For this review, take the finished solid that the model builds, in its own axes (mm). Face numbers are marked on the shaded views. A direction names the side the tool comes from. Give positions to 0.01 mm unless a question says otherwise; leave off trailing zeros. Order: outer loops, then holes, each group sorted by start corner. A loop starts at its lowest first (then second) coordinate and runs counter-clockwise, first axis right, second up.
from build123d import *

# Parameters (mm, degrees)
SKETCH_1_R               = 25
SKETCH_1_R_2             = 8
EXTRUDE_1_DEPTH          = 5
SKETCH_2_R               = 11
SKETCH_2_R_2             = 8
EXTRUDE_2_DEPTH          = 5
SKETCH_3_W               = 2
SKETCH_3_H               = 6
CUT_EXTRUDE_1_DEPTH      = 5
PATTERN_CIRCULAR_1_COUNT = 20


with BuildPart() as part:
    # 草图1 → 凸台-拉伸1 (new body)
    with BuildSketch(Plane.XY):
        Circle(SKETCH_1_R)
        Circle(SKETCH_1_R_2, mode=Mode.SUBTRACT)
    extrude(amount=EXTRUDE_1_DEPTH)

    # 草图2 → 凸台-拉伸2 (add)
    with BuildSketch(Plane.XY.offset(5)):
        Circle(SKETCH_2_R)
        Circle(SKETCH_2_R_2, mode=Mode.SUBTRACT)
    extrude(amount=EXTRUDE_2_DEPTH)

    # 草图3 → 切除-拉伸1 (cut)
    with BuildSketch(Plane.XY.offset(5)):
        with Locations((0, 19)):
            Rectangle(SKETCH_3_W, SKETCH_3_H)
    cut_extrude_1 = extrude(amount=-CUT_EXTRUDE_1_DEPTH, mode=Mode.SUBTRACT)

    # 阵列(圆周)1: 切除-拉伸1 ×20 about axis
    pattern_circular_1_axis = Axis((0, 0, 0), (0, 0, 1))
    for i in range(1, PATTERN_CIRCULAR_1_COUNT):
        add(cut_extrude_1.rotate(pattern_circular_1_axis, i * 360 / PATTERN_CIRCULAR_1_COUNT), mode=Mode.SUBTRACT)


solid = part.part
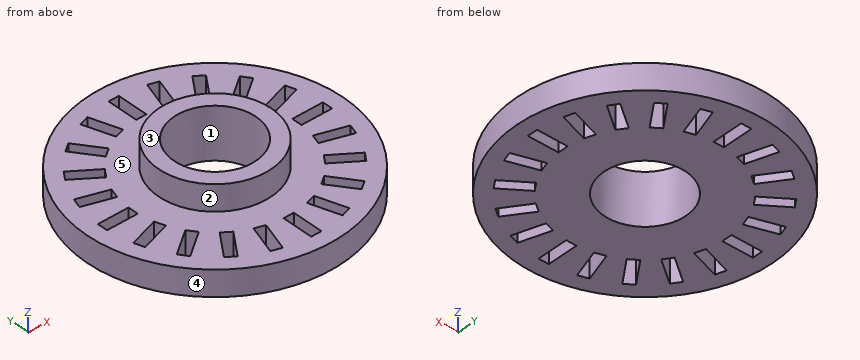
1) Draft analysis for pull direction X (two halves, no side actions). For the marked faces 1, 2 and 3, state which applies: +X half, -X half, draft (parallel to the pull), parting line (faces both ways), or undercut.
Answer sheet:
face 1: undercut
face 2: parting line
face 3: draft
2) Tool access review of the marked faces 4 and 5: name each direction out of +Z, -Z, +X, -X, +Y, -Y from which nothing blocks a thin tool from reaching the whole face with its end or side.
Answer sheet:
face 4: +Z, -Z
face 5: +Z
3) We need section A-A on y = 0. Give the boundary of the cut face in (x, z).
Answer sheet:
outline: (-25, 0) - (-22, 0) - (-22, 5) - (-25, 5) - close; (-16, 0) - (-8, 0) - (-8, 10) - (-11, 10) - (-11, 5) - (-16, 5) - close; (8, 0) - (16, 0) - (16, 5) - (11, 5) - (11, 10) - (8, 10) - close; (22, 0) - (25, 0) - (25, 5) - (22, 5) - close
4) To check wall thickness, follow line 1 (Y direction, x = 0, z = 4.75); line 2 (Y direction, x = 0, z = 7); line 3 (Y direction, x = -10, z = 4.75). State the ranges of each line that lie inside material, in increasing order.
Answer sheet:
line 1: y = -25 to -22, -16 to -8, 8 to 16, 22 to 25
line 2: y = -11 to -8, 8 to 11
line 3: y = -22.91 to -15.47, -12.51 to 12.51, 15.47 to 22.91
5) We need section C-C on z = 8.75. Give the boundary of the cut face in (x, y), then the cut area to 3 significant figures.
Answer sheet:
outline: circle Ø22 at (0, 0); hole circle Ø16 at (0, 0)
area: 179 mm2
6) Clearance check with flat-ended pins moving along their axes: pin 1 (1.5 mm diameter, centred on y = -20, z = 3, fed in from -X); pin 2 (1.6 mm diameter, centred on x = 0, z = 3, fed in from -Y); pin 3 (4 mm diameter, centred on y = 18.5, z = 2, fed in from +X). State where each tip first meets the part, or that it passes through.
Answer sheet:
pin 1: stops at x = -15.95
pin 2: stops at y = -25
pin 3: stops at x = 18.78
